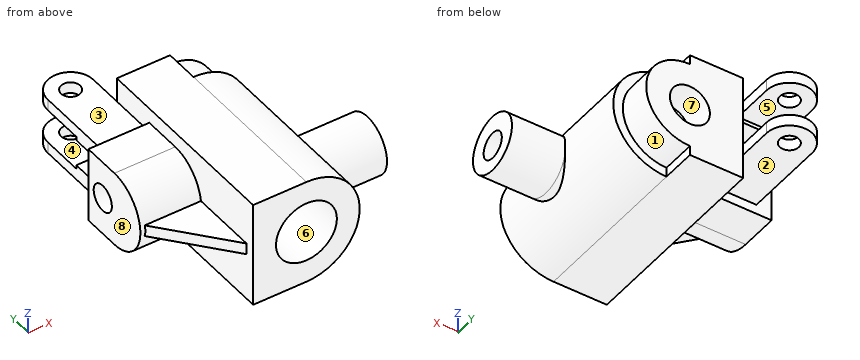
```python
from build123d import *
from build123d.topology import SkipClean

# Parameters (mm, degrees)
EXTRUDE_1_DEPTH          = 105
SKETCH_2_W               = 40
SKETCH_2_H               = 20
EXTRUDE_2_DEPTH          = 32
EXTRUDE_4_REACH          = 141.832
SKETCH_3_R               = 15
EXTRUDE_START            = 28
EXTRUDE_5_DEPTH          = 28
EXTRUDE_START_2          = 7
SKETCH_5_W               = 24
SKETCH_5_H               = 43
EXTRUDE_6_DEPTH          = 8
SKETCH_6_W               = 24
SKETCH_6_H               = 50
CUT_EXTRUDE_1_DEPTH      = 9
CUT_EXTRUDE_2_DEPTH      = 159.031642473
CUT_EXTRUDE_2_DEPTH_BACK = 159.031642473
SKETCH_7_R               = 5
RIB_1_REACH              = 156.625
SKETCH_8_WALL_W          = 356.93996261
SKETCH_8_WALL_H          = 6
CUT_EXTRUDE_START        = -18
CUT_EXTRUDE_3_DEPTH      = 18
HOLE_WIZARD_M36_2_D      = 32
HOLE_WIZARD_M36_2_DEPTH  = 55
HOLE_WIZARD_M36_2_TIP    = 9.613769904
SKETCH_14_R              = 11.5
CUT_EXTRUDE_4_DEPTH      = 78
HOLE_WIZARD_M24_1_D      = 21
HOLE_WIZARD_M24_1_DEPTH  = 16
HOLE_WIZARD_M24_1_TIP    = 6.3090365
CUT_EXTRUDE_5_DEPTH      = 130.263297345
CUT_EXTRUDE_5_DEPTH_BACK = 130.263297345
SKETCH_16_R              = 5
HOLE_WIZARD_M16_1_REACH  = 139.824
HOLE_WIZARD_M16_1_BORE_R = 7
HOLE_WIZARD_M16_2_REACH  = 157.802
HOLE_WIZARD_M16_2_BORE_R = 7


with BuildPart() as part:
    # 草图1 → 凸台-拉伸1 (new body)
    with BuildSketch(Plane(origin=(0, 0, 0), x_dir=(1, 0, 0), z_dir=(0, 1, 0))):
        with BuildLine():
            Line((-14, 28), (14, 28))
            ThreePointArc((14, 28), (42, 0), (14, -28))
            Line((14, -28), (-14, -28))
            Line((-14, -28), (-14, 28))
        make_face()
    extrude(amount=EXTRUDE_1_DEPTH)

    # 草图2 → 凸台-拉伸2 (add)
    with BuildSketch(Plane.ZY.offset(14)):
        with BuildLine():
            ThreePointArc((20, 60), (0, 40), (-20, 60))
            Line((-20, 60), (20, 60))
        make_face()
        with Locations((0, 70)):
            Rectangle(SKETCH_2_W, SKETCH_2_H)
    extrude(amount=EXTRUDE_2_DEPTH)

    # 草图3 → 凸台-拉伸4 (add, up to next)
    with BuildSketch(Plane(origin=(42, 0, 0), x_dir=(0, 0, -1), z_dir=(1, 0, 0)), mode=Mode.PRIVATE) as extrude_4_sk1:
        with Locations((0, 35)):
            Circle(SKETCH_3_R)
    extrude_4_tool1 = extrude(extrude_4_sk1.sketch, amount=-EXTRUDE_4_REACH, mode=Mode.PRIVATE) - part.part
    add(extrude_4_tool1.solids().sort_by_distance((42, 35, 0))[0])
    add(extrude_4_tool1.solids().sort_by_distance((42, 35, 0))[1])

    # 草图4 → 凸台-拉伸5 (add)
    with SkipClean():  # the faces are left unmerged after this step: merging them gives an invalid solid
        with BuildSketch(Plane(origin=(42, 0, 0), x_dir=(0, 0, -1), z_dir=(1, 0, 0)).offset(EXTRUDE_START)):
            with BuildLine():
                ThreePointArc((0, 50), (-15, 35), (0, 20))
                ThreePointArc((0, 20), (15, 35), (0, 50))
            make_face()
        extrude(amount=-EXTRUDE_5_DEPTH)

    # 草图5 → 凸台-拉伸6 (add)
    with BuildSketch(Plane.XY.offset(EXTRUDE_START_2)):
        with Locations((-26, 101.5)):
            Rectangle(SKETCH_5_W, SKETCH_5_H)
        with BuildLine():
            Line((-38, 123), (-14, 123))
            ThreePointArc((-14, 123), (-26, 135), (-38, 123))
        make_face()
    extrude_6 = extrude(amount=EXTRUDE_6_DEPTH)

    # 镜向1: 凸台-拉伸6 across plane
    add(extrude_6.mirror(Plane.XY))

    # 草图6 → 切除-拉伸1 (cut, symmetric)
    with BuildSketch(Plane.XY):
        with Locations((-26, 126)):
            Rectangle(SKETCH_6_W, SKETCH_6_H)
    extrude(amount=CUT_EXTRUDE_1_DEPTH, both=True, mode=Mode.SUBTRACT)

    # 草图7 → 切除-拉伸2 (cut, two sides: drawn at the far end of the back side and taken through both)
    with BuildSketch(Plane.XY.offset(15).offset(-CUT_EXTRUDE_2_DEPTH_BACK)):
        with Locations((-26, 123)):
            Circle(SKETCH_7_R)
    extrude(amount=CUT_EXTRUDE_2_DEPTH + CUT_EXTRUDE_2_DEPTH_BACK, mode=Mode.SUBTRACT)

    # 草图8 wall → 筋1 (add, up to next)
    with BuildSketch(Plane(origin=(-28.684243545, 22.5, 0), x_dir=(-0.642787609684, 0.766044443121, 0), z_dir=(-0.766044443121, -0.642787609684, 0)), mode=Mode.PRIVATE) as rib_1_sk1:
        Rectangle(SKETCH_8_WALL_W, SKETCH_8_WALL_H)
    rib_1_tool1 = extrude(rib_1_sk1.sketch, amount=-RIB_1_REACH, mode=Mode.PRIVATE) - part.part
    add(rib_1_tool1.solids().sort_by_distance((-28.684243545, 22.5, 0))[0])

    # 草图9 → 切除-拉伸3 (cut)
    with BuildSketch(Plane(origin=(0, 105, 0), x_dir=(1, 0, 0), z_dir=(0, 1, 0)).offset(CUT_EXTRUDE_START)):
        with BuildLine():
            Line((14, 23), (14, 28))
            ThreePointArc((14, 28), (42, 0), (14, -28))
            Line((14, -28), (14, -23))
            ThreePointArc((14, -23), (37, 0), (14, 23))
        make_face()
    extrude(amount=CUT_EXTRUDE_3_DEPTH, mode=Mode.SUBTRACT)

    # M36 螺纹孔2
    with Locations(Plane(origin=(14, 0, 0), x_dir=(0, 0, -1), z_dir=(0, -1, 0))):
        with Locations((0, 0)):
            Hole(HOLE_WIZARD_M36_2_D / 2, depth=HOLE_WIZARD_M36_2_DEPTH)
            with Locations((0, 0, -(HOLE_WIZARD_M36_2_DEPTH + HOLE_WIZARD_M36_2_TIP / 2))):  # 118° drill point
                Cone(0, HOLE_WIZARD_M36_2_D / 2, HOLE_WIZARD_M36_2_TIP, mode=Mode.SUBTRACT)

    # 草图14 → 切除-拉伸4 (cut)
    with BuildSketch(Plane.XZ):
        with Locations(Location((14, 0, 0), (0, 0, 270))):
            Circle(SKETCH_14_R)
    extrude(amount=-CUT_EXTRUDE_4_DEPTH, mode=Mode.SUBTRACT)

    # M24 螺纹孔1
    with Locations(Plane(origin=(14, 105, 0), x_dir=(0, 0, 1), z_dir=(0, 1, 0))):
        with Locations((0, 0)):
            Hole(HOLE_WIZARD_M24_1_D / 2, depth=HOLE_WIZARD_M24_1_DEPTH)
            with Locations((0, 0, -(HOLE_WIZARD_M24_1_DEPTH + HOLE_WIZARD_M24_1_TIP / 2))):  # 118° drill point
                Cone(0, HOLE_WIZARD_M24_1_D / 2, HOLE_WIZARD_M24_1_TIP, mode=Mode.SUBTRACT)

    # 草图16 → 切除-拉伸5 (cut, two sides: drawn at the far end of the back side and taken through both)
    with BuildSketch(Plane(origin=(0, 105, 0), x_dir=(1, 0, 0), z_dir=(0, 1, 0)).offset(-CUT_EXTRUDE_5_DEPTH_BACK)):
        with Locations(Location((14, 0, 0), (0, 0, 270))):
            Circle(SKETCH_16_R)
    extrude(amount=CUT_EXTRUDE_5_DEPTH + CUT_EXTRUDE_5_DEPTH_BACK, mode=Mode.SUBTRACT)

    # M16 螺纹孔1 bore (on position points) → M16 螺纹孔1 (cut, up to next)
    with BuildSketch(Plane(origin=(-46, 68.934751758, -0.063559522), x_dir=(0, 0, -1), z_dir=(-1, 0, 0)), mode=Mode.PRIVATE) as hole_wizard_m16_1_sk1:
        Circle(HOLE_WIZARD_M16_1_BORE_R)
    hole_wizard_m16_1_tool1 = extrude(hole_wizard_m16_1_sk1.sketch, amount=-HOLE_WIZARD_M16_1_REACH, mode=Mode.PRIVATE) & part.part
    add(hole_wizard_m16_1_tool1.solids().sort_by_distance((-46, 68.934752, -0.06356))[0], mode=Mode.SUBTRACT)

    # M16 螺纹孔2 bore (on position points) → M16 螺纹孔2 (cut, up to next)
    with BuildSketch(Plane(origin=(70, 35.189243523, -1.257452157), x_dir=(0, 0, 1), z_dir=(1, 0, 0)), mode=Mode.PRIVATE) as hole_wizard_m16_2_sk1:
        Circle(HOLE_WIZARD_M16_2_BORE_R)
    hole_wizard_m16_2_tool1 = extrude(hole_wizard_m16_2_sk1.sketch, amount=-HOLE_WIZARD_M16_2_REACH, mode=Mode.PRIVATE) & part.part
    add(hole_wizard_m16_2_tool1.solids().sort_by_distance((70, 35.189244, -1.257452))[0], mode=Mode.SUBTRACT)


solid = part.part
```
Work out the finished part from the listing and answer in its coordinate system (mm). Face numbers are marked on the shaded views. A direction names the side the tool comes from. Give positions to 0.01 mm unless a question says otherwise; leave off trailing zeros. Write each loop counter-clockwise with the first axis right and the second up, starting at its lowest first coordinate (ties: lowest second). Pieces come first, ordered by that corner, then holes.
(1) Flat-ended cylindrical pins translate along their axes: pin 1 Ø3 at (y, z) = (116.5, 11.5) entering from +X; pin 2 Ø2.5 at (y, z) = (92, -12) entering from -X; pin 3 Ø10 at (y, z) = (29, -1.5) entering from +X; pin 4 Ø6 at (x, y) = (-23, 67.5) entering from +Z. Find the tip coordinate at first contact, or state that the pin passes through.
Final values:
pin 1: stops at x = -14
pin 2: stops at x = -38
pin 3: stops at x = 70
pin 4: stops at z = 20
(2) The part is cut by section C-C on y = 17. Write down the section's boundary in (x, z), plus the area to 3 significant figures.
Final values:
outline: (-24.07, -3) - (-14, -3) - (-14, -28) - (14, -28) arc R28 ccw to (14, 28) - (-14, 28) - (-14, 3) - (-24.07, 3) - close; hole circle Ø32 at (14, 0)
area: 2,060 mm2
(3) Straight lines are drawn through the part: line 1 (Z direction, x = -29.5, y = 127); line 2 (Z direction, x = 14, y = 43.5); line 3 (X direction, y = 123, z = 13.6). For each, find the intervals that lie inside material, in ascending order.
Final values:
line 1: z = -15 to -9, 9 to 15
line 2: z = -28 to -16, 16 to 28
line 3: x = -38 to -31, -21 to -14
(4) The part is cut by section B-B on y = 106.5. Write down the section's boundary in (x, z), plus the area to 3 significant figures.
Final values:
outline: (-38, -15) - (-14, -15) - (-14, -9) - (-38, -9) - close; (-38, 9) - (-14, 9) - (-14, 15) - (-38, 15) - close
area: 288 mm2
(5) The part is cut by section A-A on x = -26. Count the separate pieces of the cut face and the enclosed holes in it, plus the area to 3 significant figures.
Final values:
separate pieces: 3
enclosed holes: 1
area: 2,020 mm2
(6) The mould has two halves that part along X. Classify the marked faces 5, 6, 7 and 8: pulls with the +X half, pulls with the -X half, needs draft (parallel to the pull), parting line crosses it, or undercut.
Final values:
face 5: needs draft
face 6: undercut
face 7: undercut
face 8: pulls with the -X half
(7) The part is cut by section D-D on x = 32. Write down the section's boundary in (y, z), plus the area to 3 significant figures.
Final values:
outline: (0, -21.45) - (87, -21.45) - (87, -14.32) - (105, -14.32) - (105, 14.32) - (87, 14.32) - (87, 21.45) - (0, 21.45) - close; hole circle Ø14 at (35.19, -1.26)
area: 4,090 mm2
(8) Which of the six approach directions +Z, -Z, +X, -X, +Y, -Y give full straight-line access (tool end or side, diameter ignored) to the marked faces 1, 2, 3 and 4?
Final values:
face 1: +X, +Y
face 2: -Z, -X, +Y
face 3: +Z, -X, +Y
face 4: -X, +Y
